Work out the finished part from the listing and answer in its coordinate system (mm). A direction names the side the tool comes from. Round coordinates to 2 decimals unless told otherwise and drop trailing zeros. Order: outer loops, then holes, each group sorted by start corner. A loop starts at its lowest first (then second) coordinate and runs counter-clockwise, first axis right, second up.
from build123d import *

# Parameters (mm, degrees)
SKETCH1_R           = 30.4
BOSS_EXTRUDE1_DEPTH = 260
SKETCH2_W           = 60.8
SKETCH2_H           = 35.4
BOSS_EXTRUDE2_DEPTH = 80
SKETCH3_W           = 50.8
SKETCH3_H           = 25.4
CUT_EXTRUDE1_DEPTH  = 80
CUT_EXTRUDE2_DEPTH  = 40
SKETCH5_R           = 21
CUT_EXTRUDE3_DEPTH  = 7


with BuildPart() as part:
    # Sketch1 → Boss-Extrude1 (new body)
    with BuildSketch(Plane.XY):
        Circle(SKETCH1_R)
    extrude(amount=BOSS_EXTRUDE1_DEPTH)

    # Sketch2 → Boss-Extrude2 (add)
    with BuildSketch(Plane(origin=(0, 0, 0), x_dir=(1, 0, 0), z_dir=(0, 1, 0))):
        with Locations((0, -57.7)):
            Rectangle(SKETCH2_W, SKETCH2_H)
    boss_extrude2 = extrude(amount=BOSS_EXTRUDE2_DEPTH)

    # Sketch3 → Cut-Extrude1 (cut)
    with BuildSketch(Plane(origin=(0, 80, 0), x_dir=(1, 0, 0), z_dir=(0, 1, 0))):
        with Locations((0, -57.7)):
            Rectangle(SKETCH3_W, SKETCH3_H)
    cut_extrude1 = extrude(amount=-CUT_EXTRUDE1_DEPTH, mode=Mode.SUBTRACT)

    # Mirror2: Boss-Extrude2, Cut-Extrude1 across plane
    add(boss_extrude2.mirror(Plane.XY.offset(125.4)))
    add(cut_extrude1.mirror(Plane.XY.offset(125.4)), mode=Mode.SUBTRACT)

    # Sketch4 → Cut-Extrude2 (cut)
    with BuildSketch(Plane(origin=(0, 0, 0), x_dir=(-1, 0, 0), z_dir=(0, 0, -1))):
        with BuildLine():
            Line((-3, 9.539392014), (-3, 13))
            Line((-3, 13), (3, 13))
            Line((3, 13), (3, 9.539392014))
            ThreePointArc((3, 9.539392014), (0, -10), (-3, 9.539392014))
        make_face()
    extrude(amount=-CUT_EXTRUDE2_DEPTH, mode=Mode.SUBTRACT)

    # Sketch5 → Cut-Extrude3 (cut)
    with BuildSketch(Plane.XY.offset(260)):
        Circle(SKETCH5_R)
    extrude(amount=-CUT_EXTRUDE3_DEPTH, mode=Mode.SUBTRACT)


solid = part.part
Item 1: Find section D-D (z = 159.5). Write down the section's boundary in (x, y).
Item 2: Given pin 1 (20.5 mm diameter, centred on x = -2.5, z = 194.5, fed in from +Y); pin 2 (1 mm diameter, centred on y = 11.5, z = 22.5, fed in from -X); pin 3 (2 mm diameter, centred on x = -23.5, z = 157, fed in from -Y), each flat-ended and moving along its own axis, determine where each tip first touches the part or whether it passes through.
Item 3: Find section C-C (x = 0). Write down the section's boundary in (y, z), plus the area to 3 significant figures.
Item 4: Find section B-B (z = 25). Write down the section's boundary in (x, y), plus the area to 3 significant figures.
Item 5: A tool of negligible diameter and unlimited length cuts with its end or side. For faces 4 (the face through (0, 13, 20)), 5 (the face through (25.4, 41, 58)), 6 (the face through (20, 7, 260)), from which of +Z, -Z, +X, -X, +Y, -Y can it reach the whole face along a straight path? Write none if from no direction.
Item 6: Find section A-A (y = 61). Write down the section's boundary in (x, z).
Item 7: Find the intervals of material crossed by line 1 along Z through (x, y) = (2, 73.5); line 2 along Z through (x, y) = (-17.5, 4); line 3 along X through (y, z) = (0, 21), in increasing order.
Item 8: For a pull along Y with two mould halves and no side action, classify faces 1 (the face through (-30.4, 39, 193)), 2 (the face through (0, 0, 253)), 3 (the face through (0, 80, 42)) as released by +Y, released by -Y, zero draft, split by the parting line, or undercut.
Model answer:
1. outline: circle Ø60.8 at (0, 0)
2. pin 1: stops at y = 0
2. pin 2: stops at x = -28.34
2. pin 3: stops at y = -20.44
3. outline: (-30.4, 0) - (-10, 0) - (-10, 40) - (13, 40) - (13, 0) - (30.4, 0) - (30.4, 40) - (80, 40) - (80, 45) - (0, 45) - (0, 70.4) - (80, 70.4) - (80, 75.4) - (30.4, 75.4) - (30.4, 175.4) - (80, 175.4) - (80, 180.4) - (0, 180.4) - (0, 205.8) - (80, 205.8) - (80, 210.8) - (30.4, 210.8) - (30.4, 260) - (21, 260) - (21, 253) - (-21, 253) - (-21, 260) - (-30.4, 260) - close
3. area: 14,000 mm2
4. outline: circle Ø60.8 at (0, 0); hole (-3, 9.54) arc R10 ccw (long way) to (3, 9.54) - (3, 13) - (-3, 13) - close
4. area: 2,570 mm2
5. face 4: -Z
5. face 5: +Y
5. face 6: +Z, +X, -X, +Y, -Y
6. outline: (-30.4, 40) - (30.4, 40) - (30.4, 75.4) - (-30.4, 75.4) - close; (-30.4, 175.4) - (30.4, 175.4) - (30.4, 210.8) - (-30.4, 210.8) - close; hole (-25.4, 45) - (25.4, 45) - (25.4, 70.4) - (-25.4, 70.4) - close; hole (-25.4, 180.4) - (25.4, 180.4) - (25.4, 205.8) - (-25.4, 205.8) - close
7. line 1: z = 40 to 45, 70.4 to 75.4, 175.4 to 180.4, 205.8 to 210.8
7. line 2: z = 0 to 45, 70.4 to 180.4, 205.8 to 253
7. line 3: x = -30.4 to -10, 10 to 30.4
8. face 1: zero draft
8. face 2: undercut
8. face 3: released by +Y
